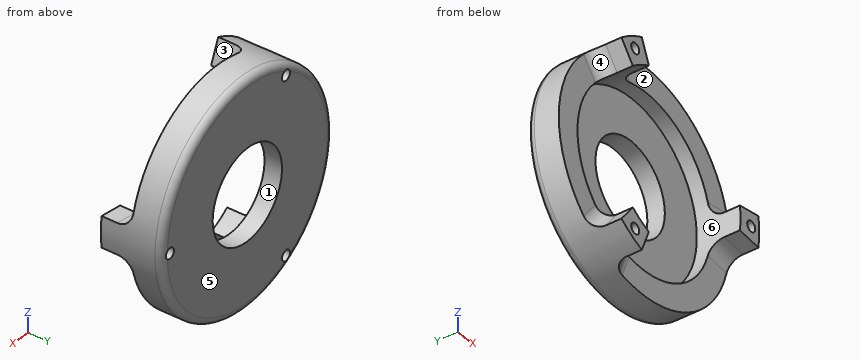
Autodesk Inventor part; units mm, degrees
ref_plane "YZ Plane" through (0, 0, 0) normal (1, 0, 0) x (0, 1, 0)
ref_plane "XZ Plane" through (0, 0, 0) normal (0, 1, 0) x (-1, 0, 0)
ref_plane "XY Plane" through (0, 0, 0) normal (0, 0, 1) x (1, 0, 0)
sketch "Sketch1" plane through (0, 0, 0) normal (0, 1, 0) x (-1, 0, 0)
  circle A0 centre (0, 0) radius 25
  circle A1 centre (0, 0) radius 32
  dimension "d0" = 50
  dimension "d1" = 64
extrude "Extrusion1" add sketch "Sketch1" along normal blind 12.5
sketch "Sketch2" plane through (0, 12.5, 0) normal (0, 1, 0) x (1, 0, 0)
  circle A0 centre (0, 0) radius 13
  circle A1 centre (0, 0) radius 32
  dimension "d4" = 26
extrude "Extrusion2" add sketch "Sketch2" along normal blind 5
sketch "Sketch4" plane through (0, 0, 0) normal (0, -1, 0) x (1, 0, 0)
  circle A0 centre (29, 0) radius 1.5
  circle A1 centre (0, 0) radius 25
  circle A2 centre (0, 0) radius 32
  dimension "d7" = 3
  dimension "d9" = 29
extrude "Extrusion3" cut sketch "Sketch4" against normal through all contours A0
pattern_circular "Circular Pattern1" count 3 over 360 about axis through (0, 0, 0) along (0, 1, 0) of "Extrusion3"
sketch "Sketch5" plane through (0, 0, 0) normal (0, -1, 0) x (1, 0, 0)
  line L0 (0, 0) -> (36.6386, -5.1024)
  line L1 (36.6386, -5.1024) -> (37.4304, -25.9892)
  line L2 (37.4304, -25.9892) -> (-15.9101, -39.2371)
  circle A0 centre (0, 0) radius 32
  line L3 (-15.9101, -39.2371) -> (0, 0)
  circle A1 centre (29, 0) radius 1.5
  circle A2 centre (-14.5, -25.1147) radius 1.5
  point P0 (-12.0246, -29.6548)
  point P1 (31.6941, -4.4138)
  dimension "d15" = 4
  dimension "d22" = 4
extrude "Extrusion4" cut sketch "Sketch5" against normal blind 8.5 contours L0 A0 L3 picked at (12.6104, -17.0364)
pattern_circular "Circular Pattern2" count 3 over 360 about axis through (0, 12.5, 0) along (0, 1, 0) of "Extrusion4"
fillet "Fillet1" radius 4 6 edges at (28.2276, 8.5, -3.931) (-10.7094, 8.5, -26.4113) (-17.5182, 8.5, -22.4803) (-17.5182, 8.5, 22.4803) (-10.7094, 8.5, 26.4113) (28.2276, 8.5, 3.931)
fillet "Fillet2" radius 2 1 edges at (-32, 17.5, 0)
properties part number "Engine retention"
Input: part model. Units: mm. Frame: model coordinates. Face numbers are marked on the shaded views. A direction names the side the tool comes from. Give positions to 0.01 mm unless a question says otherwise; leave off trailing zeros. Order: outer loops, then holes, each group sorted by start corner. A loop starts at its lowest first (then second) coordinate and runs counter-clockwise, first axis right, second up. Notation, with made-up numbers: M 39.25,16 L 87.25,16 A9 cw 87.25,29 Z; hole C 42.5,70.25 d10. An arc over 180 degrees is marked long. Answer as a JSON object with one key per item and string values.
1. Cut plane A-A, the plane y = 1. Output: boundary loops of the cut face in (x, z), and give its area (3 significant figures).
Result sheet:
{"outline": "M -19.67,-25.24 A32 ccw -12.02,-29.65 L -9.39,-23.17 A25 cw -15.37,-19.72 Z; M -19.67,25.24 L -15.37,19.72 A25 cw -9.39,23.17 L -12.02,29.65 A32 ccw Z; M 24.76,-3.45 L 31.69,-4.41 A32 ccw 31.69,4.41 L 24.76,3.45 A25 cw Z; hole C -14.5,-25.11 d3; hole C -14.5,25.11 d3; hole C 29,0 d3", "area": "144 mm²"}
2. Ray query, line 1 (X direction, y = 14.9, z = 0); line 2 (Z direction, x = 0, y = 13.65); line 3 (Z direction, x = -14, y = 12). Return the intervals inside material, ascending. Write a range as [from, to].
Result sheet:
{"line 1": "[-32, -13], [13, 27.5], [30.5, 32]", "line 2": "[-32, -13], [13, 32]", "line 3": "[-28.77, -26.53], [-23.7, -20.71], [20.71, 23.7], [26.53, 28.77]"}
3. Reachability of the marked faces 4, 5 and 6 from +Z, -Z, +X, -X, +Y, -Y: full face, straight path, thin tool, end or side. Return the list, or none.
Result sheet:
{"face 4": "-X, -Y", "face 5": "+Z, -Z, +X, -X, +Y", "face 6": "-Y"}
4. Cut plane D-D, the plane y = 13.5. Output: boundary loops of the cut face in (x, z).
Result sheet:
{"outline": "C 0,0 d64; hole C -14.5,-25.11 d3; hole C -14.5,25.11 d3; hole C 0,0 d26; hole C 29,0 d3"}
5. Pull-direction query (X, two-part tool) for the marked faces 1, 2 and 3; classes: +X half, -X half, draft (parallel to the pull), parting line (faces both ways), or undercut.
Result sheet:
{"face 1": "undercut", "face 2": "draft", "face 3": "+X half"}
6. Cut plane C-C, the plane y = 9.75. Output: boundary loops of the cut face in (x, z).
Result sheet:
{"outline": "C 0,0 d64; hole C 0,0 d50; hole C -14.5,-25.11 d3; hole C -14.5,25.11 d3; hole C 29,0 d3"}
7. First-contact query: P1, Ø1.5, axis at x = 7, y = 8.5, coming from the +Z side; P2, Ø2, axis at x = 11, y = 14.5, coming from the +Z side; P3, Ø4, axis at x = -10, y = 12.5, coming from the -Z side; P4, Ø23.5, axis at x = 0, z = 0, coming from the -Y side. Flat tips, straight axial feed; report the tip coordinate or a pass-through.
Result sheet:
{"P1": "z = 31.38", "P2": "z = 30.4", "P3": "z = -30.98", "P4": "through"}
